from build123d import *

# Parameters (mm, degrees)
SKIZZE1_W                       = 18
SKIZZE1_H                       = 10
AUFSATZ_LINEAR_AUSTRAGEN1_DEPTH = 3
DURCHGANGSLOCH_F_R_M31_D        = 3.4
SKIZZE5_W                       = 8
SKIZZE5_H                       = 3
AUFSATZ_LINEAR_AUSTRAGEN2_DEPTH = 3
AUFSATZ_LINEAR_AUSTRAGEN3_DEPTH = 10
AUFSATZ_LINEAR_AUSTRAGEN7_DEPTH = 9
SKIZZE19_W                      = 18
SKIZZE19_H                      = 3
AUFSATZ_LINEAR_AUSTRAGEN8_DEPTH = 9.2
VERRUNDUNG1_R                   = 2
VERRUNDUNG3_R                   = 2
AUFSATZ_LINEAR_AUSTRAGEN9_DEPTH = 10


with BuildPart() as part:
    # Skizze1 → Aufsatz-Linear austragen1 (new body)
    with BuildSketch(Plane.XY):
        with Locations((-9, 5)):
            Rectangle(SKIZZE1_W, SKIZZE1_H)
    extrude(amount=AUFSATZ_LINEAR_AUSTRAGEN1_DEPTH)

    # Durchgangsloch für M31 (through all)
    with Locations(Plane.XY.offset(3)):
        with Locations((-14, 0)):
            Hole(DURCHGANGSLOCH_F_R_M31_D / 2)

    # Skizze5 → Aufsatz-Linear austragen2 (add)
    with BuildSketch(Plane(origin=(0, 0, 0), x_dir=(-1, 0, 0), z_dir=(0, 0, -1))):
        with Locations((4, 1.5)):
            Rectangle(SKIZZE5_W, SKIZZE5_H)
    extrude(amount=AUFSATZ_LINEAR_AUSTRAGEN2_DEPTH)

    # Skizze7 → Aufsatz-Linear austragen3 (add)
    with BuildSketch(Plane(origin=(0, 10, 0), x_dir=(1, 0, 0), z_dir=(0, 1, 0))):
        Polygon((-6.5, -3), (-6.5, -9), (0, -9), (0, -12.2), (-9, -12.2), (-9, -3), align=None)
    extrude(amount=-AUFSATZ_LINEAR_AUSTRAGEN3_DEPTH)

    # Spiegeln2: part across plane


with BuildPart() as part_1:
    add(part.part)
    add(part.part.mirror(Plane(origin=(0, 0, 3), x_dir=(0, 0, 1), z_dir=(0, 1, 0))))

    # Skizze16 → Aufsatz-Linear austragen7 (add)
    with BuildSketch(Plane(origin=(0, 10, 0), x_dir=(1, 0, 0), z_dir=(0, 1, 0))):
        Polygon((0, 0), (-18, 0), (-18, -3), (-9, -3), (-9, -12.2), (0, -12.2), (0, -9), (-6.5, -9), (-6.5, -3), (0, -3), align=None)
    extrude(amount=AUFSATZ_LINEAR_AUSTRAGEN7_DEPTH)

    # Skizze19 → Aufsatz-Linear austragen8 (add)
    with BuildSketch(Plane.XY.offset(3)):
        with Locations((-9, 17.5)):
            Rectangle(SKIZZE19_W, SKIZZE19_H)
    extrude(amount=AUFSATZ_LINEAR_AUSTRAGEN8_DEPTH)

    # Verrundung1
    verrundung1_edges = [part_1.edges().sort_by_distance(p)[0] for p in [
        (-9, 16, 7.6),
        (-13.5, 16, 3),
        (-18, 17.5, 12.2),
        (-9, 5, 3),
    ]]
    fillet(verrundung1_edges, radius=VERRUNDUNG1_R)

    # Verrundung3
    verrundung3_edges = [part_1.edges().sort_by_distance(p)[0] for p in [
        (-18, -10, 1.5),
    ]]
    fillet(verrundung3_edges, radius=VERRUNDUNG3_R)

    # Spiegeln1: part across plane


with BuildPart() as part_2:
    add(part_1.part)
    add(part_1.part.mirror(Plane(origin=(0, 0, 3), x_dir=(0, 0, 1), z_dir=(-1, 0, 0))))

    # Skizze20 → Aufsatz-Linear austragen9 (add)
    with BuildSketch(Plane(origin=(0, 19, 0), x_dir=(1, 0, 0), z_dir=(0, 1, 0))):
        with BuildLine():
            Line((-18, 0), (-18, -10.2))
            ThreePointArc((-18, -10.2), (-17.414213562, -11.614213562), (-16, -12.2))
            Line((-16, -12.2), (16, -12.2))
            ThreePointArc((16, -12.2), (17.414213562, -11.614213562), (18, -10.2))
            Line((18, -10.2), (18, 0))
            Line((18, 0), (-18, 0))
        make_face()
    extrude(amount=AUFSATZ_LINEAR_AUSTRAGEN9_DEPTH)


solid = part_2.part
Work out the finished part from the listing and answer in its coordinate system (mm). A direction names the side the tool comes from. Round coordinates to 2 decimals unless told otherwise and drop trailing zeros. Loops run counter-clockwise (first coordinate to the right, second up) from the corner with the lowest first, then second, coordinate; pieces in that order, holes last. Notation, with made-up numbers: (6, -39) - (20, -39) arc R17 cw to (20, -9) - close; hole circle Ø8 at (-34, 54). An arc over 180 degrees is marked (long way). Use one line per item in the form item = value. Start each with the question number.
(1) Flat-ended cylindrical pins translate along their axes: P1, Ø3.5, axis at x = 16, y = -0.5, coming from the +Z side; P2, Ø2.5, axis at x = 3, z = -1.5, coming from the +Y side; P3, Ø3, axis at y = 5.5, z = 6, coming from the -X side. Find the tip coordinate at first contact, or state that the pin passes through.
(2) Determine the mould class of faces 6 (the face through (15.62, -0.51, 1.48)), 7 (the face through (-9.57, 15.4, 8.65)), 8 (the face through (0, 3, -1)) for opening direction Y: +Y half, -Y half, draft (parallel to the pull), parting line (faces both ways), or undercut.
(3) Find section B-B on x = 14. Determine the outline of the cut face in (y, z).
(4) Consider line 1 (X direction, y = 0, z = 1.9); line 2 (Y direction, x = 14, z = 1.85); line 3 (Z direction, x = 5.5, y = -5.5). Determine where each line is inside the solid, lowest interval first.
(5) Find section D-D on z = 8.5. Determine the outline of the cut face in (x, y), and give its area (3 significant figures).
(6) Which of the six approach directions +Z, -Z, +X, -X, +Y, -Y give full straight-line access (tool end or side, diameter ignored) to faces 1 (the face through (8, 0, -1)), 2 (the face through (0, 3, 9)), 3 (the face through (-15, 16, 9)), 4 (the face through (0, 0, -3)), 5 (the face through (9.6, 2.17, 3.57))?
(7) Find section C-C on x = -6. Determine the outline of the cut face in (y, z), and give its area (3 significant figures).
(8) Find section A-A on y = 0. Determine the outline of the cut face in (x, z).
Answer list:
q1.P1 = 3
q1.P2 = 3
q1.P3 = -9.06
q2.face_6 = undercut
q2.face_7 = -Y half
q2.face_8 = +Y half
q3.outline = (-10, 0) - (-1.7, 0) - (-1.7, 3) - (-10, 3) - close; (1.7, 0) - (29, 0) - (29, 12.2) - (16, 12.2) - (16, 5) arc R2 cw to (14, 3) - (1.7, 3) - close
q4.line_1 = -18 to -15.7, -12.3 to 12.3, 15.7 to 18
q4.line_2 = -10 to -1.7, 1.7 to 29
q4.line_3 = 0 to 3, 9 to 12.2
q5.outline = (-18, 16) - (-11, 16) arc R2 cw to (-9, 14) - (-9, -10) - (-6.5, -10) - (-6.5, 16) - (6.5, 16) - (6.5, -10) - (9, -10) - (9, 14) arc R2 cw to (11, 16) - (18, 16) - (18, 29) - (-18, 29) - close
q5.area = 600 mm^2
q6.face_1 = -Z, +X, +Y, -Y
q6.face_2 = -Y
q6.face_3 = +Z, -X, -Y
q6.face_4 = -Z, +X, -X, +Y, -Y
q6.face_5 = +Z, +X, -Y
q7.outline = (-10, 0) - (-3, 0) - (-3, -3) - (3, -3) - (3, 0) - (29, 0) - (29, 12.2) - (-10, 12.2) - (-10, 9) - (16, 9) - (16, 3) - (-10, 3) - close
q7.area = 338 mm^2
q8.outline = (-18, 0) - (-15.7, 0) - (-15.7, 3) - (-18, 3) - close; (-12.3, 0) - (-8, 0) - (-8, -3) - (8, -3) - (8, 0) - (12.3, 0) - (12.3, 3) - (11, 3) arc R2 cw to (9, 5) - (9, 12.2) - (-9, 12.2) - (-9, 5) arc R2 cw to (-11, 3) - (-12.3, 3) - close; (15.7, 0) - (18, 0) - (18, 3) - (15.7, 3) - close; hole (-6.5, 3) - (6.5, 3) - (6.5, 9) - (-6.5, 9) - close
